The listing builds one solid part. Answer for the finished solid, in the listing's coordinates (mm). A direction names the side the tool comes from. Give positions to 0.01 mm unless a question says otherwise; leave off trailing zeros. Loops run counter-clockwise (first coordinate to the right, second up) from the corner with the lowest first, then second, coordinate; pieces in that order, holes last. Notation, with made-up numbers: (-14, -29) - (33, -29) arc R6 cw to (33, -24) - close; hole circle Ø11 at (4, 49). An arc over 180 degrees is marked (long way). Write item = value, one per line. Start each with the question number.
1) Which of the six approach directions +Z, -Z, +X, -X, +Y, -Y give full straight-line access (tool end or side, diameter ignored) to faces 4 (the flat face through (16, 7.5, 9)), 5 (the flat face through (8, -13.873, 7)), 6 (the flat face through (10.5, 4.4, 9)), 7 (the cylindrical face through (1.285, -23.599, 7.605)), 8 (the flat face through (16, -7.5, 9))?
2) The part is cut by section C-C on y = -18.5. Write down the section's boundary in (x, z).
3) The mould has two halves that part along Y. Classify faces 1 (the cylindrical face through (-6.67, -14.58, 10.54)), 2 (the cylindrical face through (-8.847, -23.599, 7.395)), 3 (the flat face through (-9.132, -13, 8)): +Y half, -Y half, draft (parallel to the pull), parting line (faces both ways), or undercut.
4) The part is cut by section B-B on x = 4.5. Write down the section's boundary in (y, z), plus the area to 3 significant figures.
5) The part is cut by section D-D on y = -5.5. Write down the section's boundary in (x, z), plus the area to 3 significant figures.
6) The part is cut by section A-A on y = 0. Write down the section's boundary in (x, z), plus the area to 3 significant figures.
7) Flat-ended cylindrical pins translate along their axes: P1, Ø1, axis at x = -9, z = 8, coming from the -Y side; P2, Ø1.5, axis at y = 3, z = 8, coming from the -X side; P3, Ø8.5, axis at y = -17, z = 9.5, coming from the -X side; P4, Ø4, axis at x = 16, y = 0, coming from the -Z side. Find the tip coordinate at first contact, or state that the pin passes through.
8) Consider probe 1 along X at (y, z) = (-18.5, 2); probe 2 along Y at (x, z) = (6, 8.75); probe 3 along Z at (x, y) = (17.85, 0). Determine where each line is inside the solid, lowest interval first.
from build123d import *

# Parameters (mm, degrees)
SKETCH_R        = 15
PAD_DEPTH       = 15
SKETCH001_R     = 11.2
POCKET_DEPTH    = 15.001
SKETCH002_W     = 8
SKETCH002_H     = 15
PAD001_DEPTH    = 12
SKETCH003_W     = 18.264062
SKETCH003_H     = 12
PAD002_DEPTH    = 15
SKETCH004_R     = 2.8
POCKET001_DEPTH = 30.133031
POCKET002_DEPTH = 3
SKETCH006_R     = 4.5
POCKET003_DEPTH = 5
SKETCH007_W     = 2
SKETCH007_H     = 28.949347
POCKET004_DEPTH = 15.001
POCKET005_DEPTH = 2.5
SKETCH008_R     = 2.8
POCKET006_DEPTH = 14
FILLET_R        = 1
FILLET001_R     = 1


with BuildPart() as part:
    # Sketch → Pad (new body)
    with BuildSketch(Plane.XY):
        Circle(SKETCH_R)
    extrude(amount=PAD_DEPTH)

    # Sketch001 → Pocket (cut, through all)
    with BuildSketch(Plane.XY.offset(15)):
        Circle(SKETCH001_R)
    extrude(amount=-POCKET_DEPTH, mode=Mode.SUBTRACT)

    # Sketch002 → Pad001 (new body)
    with BuildSketch(Plane.XY.offset(15)):
        with Locations((17, 0)):
            Rectangle(SKETCH002_W, SKETCH002_H)
    extrude(amount=-PAD001_DEPTH)

    # Sketch003 → Pad002 (new body)
    with BuildSketch(Plane.XY.offset(15)):
        with Locations((0, -17.899832)):
            Rectangle(SKETCH003_W, SKETCH003_H)
    extrude(amount=-PAD002_DEPTH)

    # Sketch004 → Pocket001 (cut, through all)
    with BuildSketch(Plane(origin=(-9.132031, 0, 0), x_dir=(0, -1, 0), z_dir=(-1, 0, 0))):
        with Locations((17.899832, 7.5)):
            Circle(SKETCH004_R)
    extrude(amount=-POCKET001_DEPTH, mode=Mode.SUBTRACT)

    # Sketch005 → Pocket002 (cut)
    with BuildSketch(Plane.YZ.offset(9.132031)):
        Polygon((-18.023397, 2.63711), (-13.873397, 5.033113), (-13.873397, 9.825121), (-18.023397, 12.221124), (-22.173397, 9.825121), (-22.173397, 5.033113), align=None)
    extrude(amount=-POCKET002_DEPTH, mode=Mode.SUBTRACT)

    # Sketch006 → Pocket003 (cut)
    with BuildSketch(Plane(origin=(-9.132031, 0, 0), x_dir=(0, -1, 0), z_dir=(-1, 0, 0))):
        with Locations((17.899832, 7.5)):
            Circle(SKETCH006_R)
    extrude(amount=-POCKET003_DEPTH, mode=Mode.SUBTRACT)

    # Sketch007 → Pocket004 (cut, through all)
    with BuildSketch(Plane.XY.offset(15)):
        with Locations((0, -19.659897)):
            Rectangle(SKETCH007_W, SKETCH007_H)
    extrude(amount=-POCKET004_DEPTH, mode=Mode.SUBTRACT)

    # Sketch009 → Pocket005 (cut, symmetric)
    with BuildSketch(Plane(origin=(13, 0, 0), x_dir=(0, -1, 0), z_dir=(-1, 0, 0))):
        Polygon((2.396004, 4.85), (4.792007, 9), (2.396004, 13.15), (-2.396004, 13.15), (-4.792007, 9), (-2.396004, 4.85), align=None)
    extrude(amount=POCKET005_DEPTH, both=True, mode=Mode.SUBTRACT)

    # Sketch008 → Pocket006 (cut)
    with BuildSketch(Plane.YZ.offset(21)):
        with Locations((0, 9)):
            Circle(SKETCH008_R)
    extrude(amount=-POCKET006_DEPTH, mode=Mode.SUBTRACT)

    # Fillet
    fillet_edges = [part.edges().sort_by_distance(p)[0] for p in [
        (21, 7.5, 9),
        (21, -7.5, 9),
        (9.132031, -23.899832, 7.5),
        (1, -23.899832, 7.5),
        (-1, -23.899832, 7.5),
        (-9.132031, -23.899832, 7.5),
    ]]
    fillet(fillet_edges, radius=FILLET_R)

    # Fillet001
    fillet001_edges = [part.edges().sort_by_distance(p)[0] for p in [
        (1, -11.155268, 7.5),
        (-1, -11.155268, 7.5),
    ]]
    fillet(fillet001_edges, radius=FILLET001_R)


solid = part.part
Answer below:
q1.face_4 = +Z, -Z, +X, +Y
q1.face_5 = +X
q1.face_6 = none
q1.face_7 = +Z, -Z, -Y
q1.face_8 = +Z, -Z, +X, -Y
q2.outline = (-9.13, 0) - (-1, 0) - (-1, 4.77) - (-4.13, 4.77) - (-4.13, 3.04) - (-9.13, 3.04) - close; (-9.13, 11.96) - (-4.13, 11.96) - (-4.13, 10.23) - (-1, 10.23) - (-1, 15) - (-9.13, 15) - close; (1, 0) - (9.13, 0) - (9.13, 2.91) - (6.13, 2.91) - (6.13, 4.77) - (1, 4.77) - close; (1, 10.23) - (6.13, 10.23) - (6.13, 11.95) - (9.13, 11.95) - (9.13, 15) - (1, 15) - close
q3.face_1 = undercut
q3.face_2 = -Y half
q3.face_3 = draft
q4.outline = (-23.9, 0) - (-10.26, 0) - (-10.26, 15) - (-23.9, 15) - close; (10.26, 0) - (14.31, 0) - (14.31, 15) - (10.26, 15) - close; hole circle Ø5.6 at (-17.9, 7.5)
q4.area = 241 mm2
q5.outline = (-13.96, 0) - (-9.76, 0) - (-9.76, 15) - (-13.96, 15) - close; (9.76, 0) - (13.96, 0) - (13.96, 3) - (21, 3) - (21, 15) - (9.76, 15) - close
q5.area = 210 mm2
q6.outline = (-15, 0) - (-11.2, 0) - (-11.2, 15) - (-15, 15) - close; (11.2, 0) - (15, 0) - (15, 3) - (21, 3) - (21, 6.2) - (15.5, 6.2) - (15.5, 4.85) - (11.2, 4.85) - close; (11.2, 13.15) - (15.5, 13.15) - (15.5, 11.8) - (21, 11.8) - (21, 15) - (11.2, 15) - close
q6.area = 120 mm2
q7.P1 = -23.83
q7.P2 = -14.83
q7.P3 = -9.13
q7.P4 = 0
q8.probe_1 = -9.13 to -1, 1 to 9.13
q8.probe_2 = -23.9 to -20.41, -15.39 to -9.46, 9.46 to 13.75
q8.probe_3 = 3 to 6.2, 11.8 to 15
